For this review, take the finished solid that the model builds, in its own axes (mm). Round coordinates to 2 decimals unless told otherwise and drop trailing zeros. Loops run counter-clockwise (first coordinate to the right, second up) from the corner with the lowest first, then second, coordinate; pieces in that order, holes last.
1. To check wall thickness, follow line 1 along Y through (x, z) = (162, 4); line 2 along Y through (x, z) = (291, 0.25); line 3 along X through (y, z) = (-119, -0.5). State the ranges of each line that lie inside material, in increasing order.
2. Consider section B-B on x = 35.5. State the section outline as (y, z) points.
3. Clearance check with flat-ended pins moving along their axes: pin 1 Ø5 at (x, y) = (292, 161) entering from +Z; pin 2 Ø1 at (x, z) = (74, -1) entering from -Y; pin 3 Ø2 at (y, z) = (48.5, -1) entering from +X. State where each tip first meets the part, or that it passes through.
4. Consider section A-A on z = 0. State the section outline as (x, y) points.
5. Consider section D-D on y = 0. State the section outline as (x, z) points.
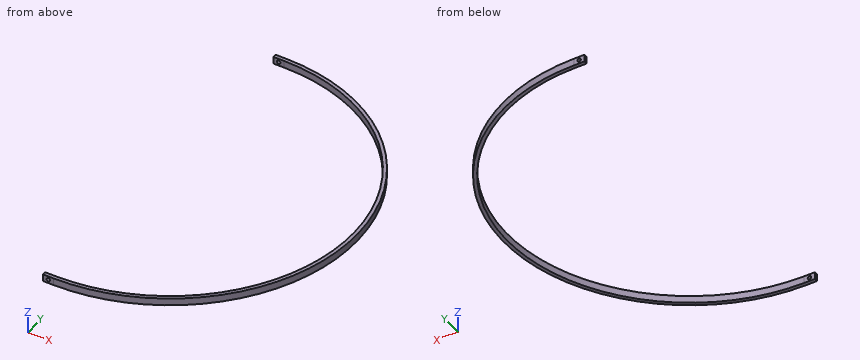
from build123d import *

# Parameters (mm, degrees)
SKETCH1_W           = 12.7
SKETCH1_H           = 6.35
BOSS_EXTRUDE1_DEPTH = 19.05
SKETCH2_R           = 3.175
CUT_EXTRUDE1_DEPTH  = 19.05
SKETCH9_W           = 12.7
SKETCH9_H           = 6.35
REVOLVE1_ANGLE      = 90


with BuildPart() as part:
    # Sketch1 → Boss-Extrude1 (new body)
    with BuildSketch(Plane(origin=(0, 0, 0), x_dir=(0, 0, -1), z_dir=(1, 0, 0))):
        with Locations((0, 327.025)):
            Rectangle(SKETCH1_W, SKETCH1_H)
    extrude(amount=-BOSS_EXTRUDE1_DEPTH)

    # Sketch2 → Cut-Extrude1 (cut)
    with BuildSketch(Plane(origin=(0, 330.2, 0), x_dir=(1, 0, 0), z_dir=(0, 1, 0))):
        with Locations(Location((-9.525, 0, 0), (0, 0, 270))):
            Circle(SKETCH2_R)
    extrude(amount=-CUT_EXTRUDE1_DEPTH, mode=Mode.SUBTRACT)

    # Sketch9 → Revolve1 (revolve)
    with BuildSketch(Plane(origin=(0, 0, 0), x_dir=(0, 0, -1), z_dir=(1, 0, 0))):
        with Locations((0, 327.025)):
            Rectangle(SKETCH9_W, SKETCH9_H)
    revolve(axis=Axis((0, 0, -195.31411855), (0, 0, -1)), revolution_arc=REVOLVE1_ANGLE)

    # Mirror2: part across plane


with BuildPart() as part_1:
    add(part.part)
    add(part.part.mirror(Plane.ZX))


solid = part_1.part
Resolved:
1. line 1: y = -287.73 to -280.42, 280.42 to 287.73
1. line 2: y = -156.05 to -142.12, 142.12 to 156.05
1. line 3: x = 301.19 to 308.01
2. outline: (-328.29, -6.35) - (-321.9, -6.35) - (-321.9, 6.35) - (-328.29, 6.35) - close; (321.9, -6.35) - (328.29, -6.35) - (328.29, 6.35) - (321.9, 6.35) - close
3. pin 1: passes through
3. pin 2: stops at y = -321.92
3. pin 3: stops at x = 326.77
4. outline: (-19.05, -330.2) - (-12.7, -330.2) - (-12.7, -323.85) - (-19.05, -323.85) - close; (-19.05, 323.85) - (-12.7, 323.85) - (-12.7, 330.2) - (-19.05, 330.2) - close; (-6.35, -330.2) - (0, -330.2) arc R330.2 ccw to (0, 330.2) - (-6.35, 330.2) - (-6.35, 323.85) - (0, 323.85) arc R323.85 cw to (0, -323.85) - (-6.35, -323.85) - close
5. outline: (323.85, -6.35) - (330.2, -6.35) - (330.2, 6.35) - (323.85, 6.35) - close
